Study the drawing (mm; zero at the part's minimum x, y, z) and answer. A direction names the side the tool comes from. Coordinates: 2 decimals unless noted, no trailing zeros. Order: outer loops, then holes, each group sorted by start corner. A loop starts at its lowest first (then second) coordinate and runs counter-clockwise, first axis right, second up.
1. The part is cut by section A-A, the plane x = 43. Give the vertices of the cut face in (y, z).
2. The part is cut by section D-D, the plane x = 7. Give the vertices of the cut face in (y, z), then the cut area to 4 significant figures.
3. A tool of negligible diameter and unlimited length cuts with its end or side. For the marked faces 4, 5 and 6, from which of +Z, -Z, +X, -X, +Y, -Y can it reach the whole face along a straight path? Write none if from no direction.
4. The part is cut by section B-B, the plane z = 31.5. Give the vertices of the cut face in (x, y).
5. Flat-ended cylindrical pins translate along their axes: pin 1 Ø3 at (x, y) = (72.5, 10) entering from +Z; pin 2 Ø3.5 at (x, y) = (76.5, 6) entering from +Z; pin 3 Ø3 at (x, y) = (48.75, 9) entering from -Z; pin 4 Ø1.5 at (x, y) = (42, 3) entering from -Z. Find the tip coordinate at first contact, or state that the pin passes through.
6. Find the intervals of material crossed by probe 1 along X at (y, z) = (13.25, 15); probe 2 along X at (y, z) = (5, 4.5); probe 3 along Y at (x, z) = (48.75, 42.95), in increasing order.
7. Determine the mould class of the marked faces 1, 2 and 3 for opening direction X: +X half, -X half, draft (parallel to the pull), parting line (faces both ways), or undercut.
8. The part is cut by section C-C, the plane y = 9. Count the separate pieces of the cut face and the enclosed holes in it, then the cut area to 4 significant figures.
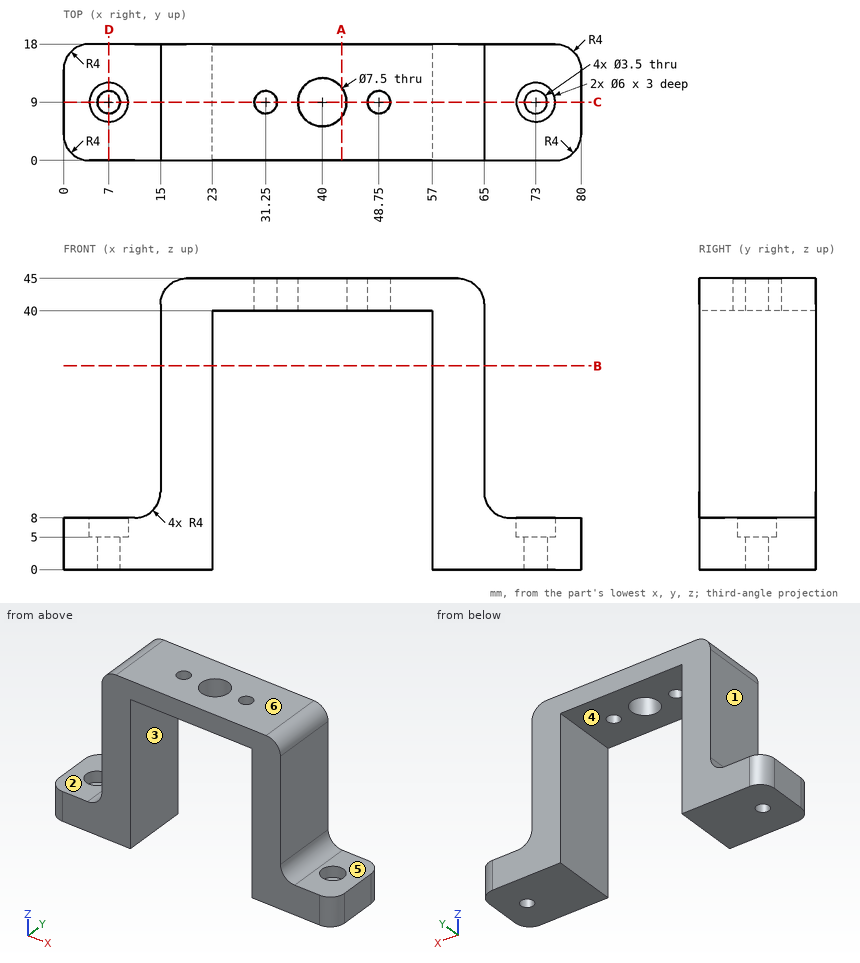
Geometry says:
1. outline: (0, 40) - (6.75, 40) - (6.75, 45) - (0, 45) - close; (11.25, 40) - (18, 40) - (18, 45) - (11.25, 45) - close
2. outline: (0, 0) - (7.25, 0) - (7.25, 5) - (6, 5) - (6, 8) - (0, 8) - close; (10.75, 0) - (18, 0) - (18, 8) - (12, 8) - (12, 5) - (10.75, 5) - close
2. area: 108.5 mm2
3. face 4: -Z, +Y, -Y
3. face 5: +Z, +X, +Y, -Y
3. face 6: +Z, +X, -X, +Y, -Y
4. outline: (15, 0) - (23, 0) - (23, 18) - (15, 18) - close; (57, 0) - (65, 0) - (65, 18) - (57, 18) - close
5. pin 1: stops at z = 5
5. pin 2: stops at z = 8
5. pin 3: passes through
5. pin 4: stops at z = 40
6. probe 1: x = 15 to 23, 57 to 65
6. probe 2: x = 0 to 23, 57 to 80
6. probe 3: y = 0 to 7.25, 10.75 to 18
7. face 1: -X half
7. face 2: draft
7. face 3: undercut
8. separate pieces: 6
8. enclosed holes: 0
8. area: 986.5 mm2
